Could you check a few things on this model? Use its own coordinates, in mm. Round coordinates to 2 decimals unless told otherwise and drop trailing zeros. Write each loop counter-clockwise with the first axis right and the second up, starting at its lowest first coordinate (ties: lowest second). Pieces come first, ordered by that corner, then holes. Notation, with made-up numbers: M 6,-28.75 L 49,-28.75 A17 ccw 49,-14.75 Z; hole C -38,6 d5. An arc over 180 degrees is marked long. One line per item, written item: value. Start each with the question number.
(1) If I drill on L1, parallel to Y at x = -38.5, z = 1.5; L2, parallel to X at y = 26, z = 2.9; L3, parallel to X at y = -3, z = 0.7, over which ranges is the centre line in solid material (lowest first)?
(2) I want a section at D-D on y = 12. Please give me the cut outline in (x, z), and give its area (3 significant figures).
(3) I want a section at C-C on z = 2.5. Count the separate pieces of the cut face and the enclosed holes in it, and give its area (3 significant figures).
(4) I'm going to push flat-ended pins straight in: pin 1 Ø3.5 at (x, y) = (-50.5, 0) entering from +Z (1 decimal); pin 2 Ø1 at (y, z) = (10.5, 4) entering from -X. Where does each tip first touch, or does it pass through?
(5) I want a section at A-A on y = -12. Please give me the cut outline in (x, z), and give its area (3 significant figures).
(6) I want a section at B-B on x = -61. Please give me the cut outline in (y, z), and give its area (3 significant figures).
```python
from build123d import *

# Parameters (mm, degrees)
SKETCH1_R           = 4
SKETCH1_R_2         = 5
SKETCH1_R_3         = 2.5
SKETCH1_R_4         = 2
SKETCH1_R_5         = 1.5
BOSS_EXTRUDE1_DEPTH = 5


with BuildPart() as part:
    # Sketch1 → Boss-Extrude1 (new body)
    with BuildSketch(Plane.XY):
        with BuildLine():
            Line((-38.5, 32.5), (38.5, 32.5))
            ThreePointArc((38.5, 32.5), (71, 0), (38.5, -32.5))
            Line((38.5, -32.5), (-38.5, -32.5))
            ThreePointArc((-38.5, -32.5), (-71, 0), (-38.5, 32.5))
        make_face()
        with Locations((-38.5, 0)):
            Circle(SKETCH1_R, mode=Mode.SUBTRACT)
        with Locations((38.5, 0)):
            Circle(SKETCH1_R_2, mode=Mode.SUBTRACT)
        with Locations((20.25, 0)):
            Circle(SKETCH1_R_3, mode=Mode.SUBTRACT)
        with Locations((56.75, 0)):
            Circle(SKETCH1_R_3, mode=Mode.SUBTRACT)
        with Locations((-38.5, -12)):
            Circle(SKETCH1_R_4, mode=Mode.SUBTRACT)
        with Locations((-26.5, 0)):
            Circle(SKETCH1_R_4, mode=Mode.SUBTRACT)
        with Locations((-38.5, 12)):
            Circle(SKETCH1_R_4, mode=Mode.SUBTRACT)
        with Locations((-50.5, 0)):
            Circle(SKETCH1_R_4, mode=Mode.SUBTRACT)
        with Locations((-38.5, 22.5)):
            Circle(SKETCH1_R_5, mode=Mode.SUBTRACT)
        with Locations((-16, 0)):
            Circle(SKETCH1_R_5, mode=Mode.SUBTRACT)
        with Locations((-38.5, -22.5)):
            Circle(SKETCH1_R_5, mode=Mode.SUBTRACT)
        with Locations((-61, 0)):
            Circle(SKETCH1_R_5, mode=Mode.SUBTRACT)
        with Locations((11.5, 0)):
            Circle(SKETCH1_R_5, mode=Mode.SUBTRACT)
        with Locations((11.5, -25)):
            Circle(SKETCH1_R_5, mode=Mode.SUBTRACT)
        with Locations((11.5, 25)):
            Circle(SKETCH1_R_5, mode=Mode.SUBTRACT)
        with Locations((45.81132848, 24.189554469)):
            Circle(SKETCH1_R_5, mode=Mode.SUBTRACT)
        with Locations((45.416389416, 17.200704553)):
            Circle(SKETCH1_R_5, mode=Mode.SUBTRACT)
        Polygon((42.503089082, 27.681767532), (41.735778899, 14.103430555), (34.796849341, 14.495548626), (35.564159523, 28.073885604), align=None, mode=Mode.SUBTRACT)
        with BuildLine():
            ThreePointArc((-0.320277112, -17.501678783), (0.172057271, -18.827426442), (1.49780493, -18.335092058))
            ThreePointArc((1.49780493, -18.335092058), (3.434628419, -13.322422428), (4.745938398, -8.111030272))
            ThreePointArc((4.745938398, -8.111030272), (3.947417759, -6.943826439), (2.780213925, -7.742347078))
            ThreePointArc((2.780213925, -7.742347078), (1.528508946, -12.716857772), (-0.320277112, -17.501678783))
        make_face(mode=Mode.SUBTRACT)
    extrude(amount=BOSS_EXTRUDE1_DEPTH)


solid = part.part
```
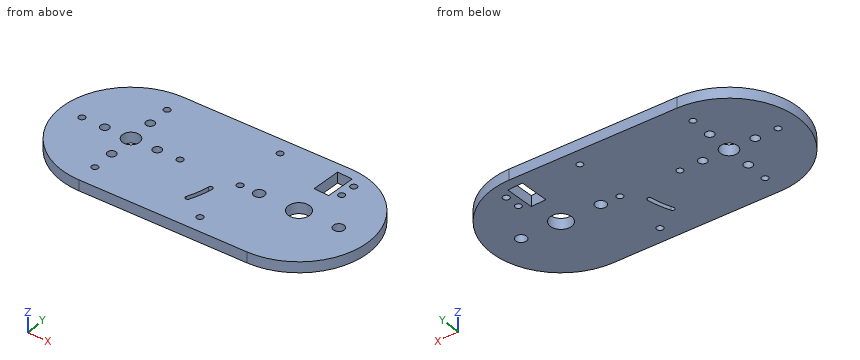
Found:
1. L1: y = -32.5 to -24, -21 to -14, -10 to -4, 4 to 10, 14 to 21, 24 to 32.5
1. L2: x = -58 to 10.38, 12.62 to 35.45, 42.41 to 58
1. L3: x = -70.86 to -41.15, -35.85 to 34.5, 42.5 to 70.86
2. outline: M -68.7,0 L -40.5,0 L -40.5,5 L -68.7,5 Z; M -36.5,0 L 68.7,0 L 68.7,5 L -36.5,5 Z
2. area: 667 mm²
3. separate pieces: 1
3. enclosed holes: 19
3. area: 7,920 mm²
4. pin 1: passes through
4. pin 2: stops at x = -69.42
5. outline: M -68.7,0 L -40.5,0 L -40.5,5 L -68.7,5 Z; M -36.5,0 L 1.75,0 L 1.75,5 L -36.5,5 Z; M 3.83,0 L 68.7,0 L 68.7,5 L 3.83,5 Z
5. area: 657 mm²
6. outline: M -23.45,0 L -1.5,0 L -1.5,5 L -23.45,5 Z; M 1.5,0 L 23.45,0 L 23.45,5 L 1.5,5 Z
6. area: 220 mm²
